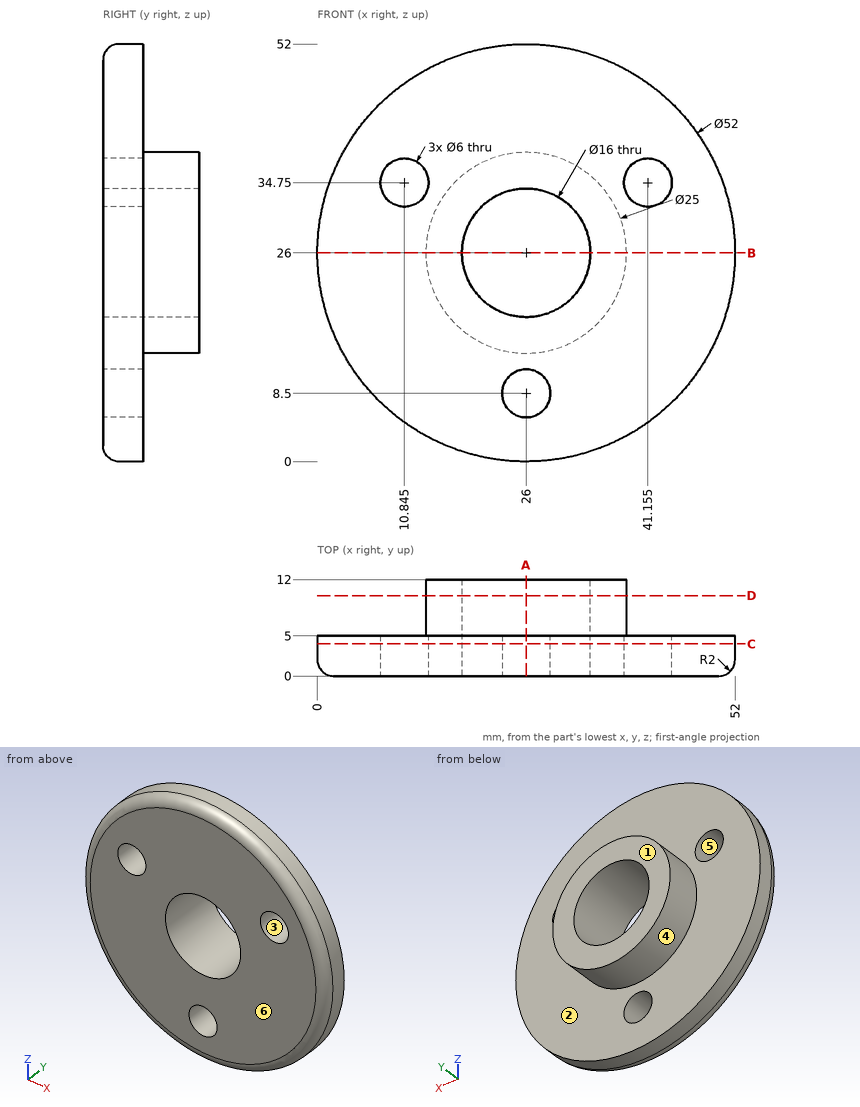
Answer from the drawing. Dimensions are ordinates in mm from the lowest x, y and z of the part. A direction names the side the tool comes from. Give positions to 0.01 mm unless a question says otherwise; leave off trailing zeros. Order: outer loops, then holes, each group sorted by start corner. A loop starts at its lowest first (then second) coordinate and runs counter-clockwise, first axis right, second up.
(1) Find section B-B (z = 26). Give the vertices of the cut face in (x, y), plus the area to 3 significant figures.
(2) Find section C-C (y = 4). Give the number of separate pieces and of enclosed holes in the cut face, plus the area to 3 significant figures.
(3) For a pull along X with two mould halves and no side action, classify the marked faces 3, 4, 5 and 6 as released by +X, released by -X, zero draft, split by the parting line, or undercut.
(4) For the marked faces 1 and 2, determine the directions among +Z, -Z, +X, -X, +Y, -Y from which every point of the face is accessible in a straight line to the end or side of a thin tool.
(5) Find section D-D (y = 10). Give the vertices of the cut face in (x, z), plus the area to 3 significant figures.
(6) Straight lines are drawn through the part: L1, parallel to Z at x = 26, y = 3.55; L2, parallel to X at y = 3, z = 26; L3, parallel to X at y = 2.85, z = 34.75 (1 decimal). For each, find the intervals that lie inside material, in ascending order.
(7) Find section A-A (x = 26). Give the vertices of the cut face in (y, z).
(8) Given pin 1 (1.5 mm diameter, centred on x = 25.5, y = 5.5, fed in from -Z); pin 2 (1.5 mm diameter, centred on x = 8.5, z = 40, fed in from -Y); pin 3 (8 mm diameter, centred on x = 41.16, z = 34.75, fed in from +Y); pin 4 (5 mm diameter, centred on y = 9, z = 34, fed in from -X) (1 decimal), each flat-ended and moving along its own axis, determine where each tip first touches the part or whether it passes through.
Result sheet:
1. outline: (0, 2) arc R2 ccw to (2, 0) - (18, 0) - (18, 12) - (13.5, 12) - (13.5, 5) - (0, 5) - close; (34, 0) - (50, 0) arc R2 ccw to (52, 2) - (52, 5) - (38.5, 5) - (38.5, 12) - (34, 12) - close
1. area: 241 mm2
2. separate pieces: 1
2. enclosed holes: 4
2. area: 1,840 mm2
3. face 3: undercut
3. face 4: split by the parting line
3. face 5: undercut
3. face 6: zero draft
4. face 1: +Z, -Z, +X, -X, +Y
4. face 2: +Y
5. outline: circle Ø25 at (26, 26); hole circle Ø16 at (26, 26)
5. area: 290 mm2
6. L1: z = 0 to 5.5, 11.5 to 18, 34 to 52
6. L2: x = 0 to 18, 34 to 52
6. L3: x = 1.5 to 7.8, 13.8 to 38.2, 44.2 to 50.5
7. outline: (0, 2) arc R2 ccw to (2, 0) - (5, 0) - (5, 5.5) - (0, 5.5) - close; (0, 11.5) - (5, 11.5) - (5, 13.5) - (12, 13.5) - (12, 18) - (0, 18) - close; (0, 34) - (12, 34) - (12, 38.5) - (5, 38.5) - (5, 52) - (2, 52) arc R2 ccw to (0, 50) - close
8. pin 1: stops at z = 0
8. pin 2: stops at y = 0
8. pin 3: stops at y = 5
8. pin 4: stops at x = 14.8
